from build123d import *

# Parameters (mm, degrees)
EXTRUDE_1_DEPTH = 75
CHAMFER_1_SIZE  = 15
CHAMFER_2_SIZE  = 3


with BuildPart() as part:
    # 草图1 → 凸台-拉伸1 (new body)
    with BuildSketch(Plane.XY):
        Polygon((0, 0), (70, 0), (70, 5), (40, 5), (40, 55), (37, 55), (37, 5), (35.2, 5), (35.2, 55), (32.2, 55), (32.2, 5), (0, 5), align=None)
    extrude(amount=EXTRUDE_1_DEPTH)

    # 倒角1
    chamfer_1_edges = [part.edges().sort_by_distance(p)[0] for p in [
        (32.2, 5, 37.5),
        (40, 5, 37.5),
    ]]
    chamfer(chamfer_1_edges, length=CHAMFER_1_SIZE)

    # 倒角2
    chamfer_2_edges = [part.edges().sort_by_distance(p)[0] for p in [
        (37, 55, 37.5),
        (35.2, 55, 37.5),
    ]]
    chamfer(chamfer_2_edges, length=CHAMFER_2_SIZE - 0.0001)  # a hair under: the kernel refuses the full size


solid = part.part
CAD build for the part. Positions are in the model's coordinates, mm. A direction names the side the tool comes from. Coordinates: 2 decimals unless noted, no trailing zeros. Write each loop counter-clockwise with the first axis right and the second up, starting at its lowest first coordinate (ties: lowest second). Pieces come first, ordered by that corner, then holes. Notation, with made-up numbers: M 23.5,-2.75 L 56.5,-2.75 A30 ccw 56.5,24.25 Z; hole C -35.5,-12.5 d11. An arc over 180 degrees is marked long. Answer as a JSON object with one key per item and string values. Group by question number.
1) Saw through at C-C (x = 62.5). Write the cut outline in (y, z).
2) Mould opens along X. For faces 1 (the face through (0, 3, 37)), 2 (the face through (35.2, 28, 37)), 3 (the face through (35, 17, 75)), 4 (the face through (37, 29, 37)) say: +X half, -X half, draft (parallel to the pull), parting line (faces both ways), or undercut.
3) Saw through at A-A (y = 15.5). Write the cut outline in (x, z), plus the area to 4 significant figures.
4) Pin check, flat tips, straight feed: pin 1 Ø4 at (x, z) = (28.5, 31) entering from +Y; pin 2 Ø5 at (x, z) = (6.5, 49.5) entering from +Y; pin 3 Ø3 at (y, z) = (44, 12.5) entering from +X. Stop position of each tip, or through.
5) Saw through at D-D (y = 6). Write the cut outline in (x, z).
6) Tool access for faces 5 (the face through (32.2, 38, 37)), 6 (the face through (33.7, 53.5, 37)), 7 (the face through (35, 17, 0)), 8 (the face through (40, 37, 37)), 9 (the face through (35, 0, 37)): list every direction of +Z, -Z, +X, -X, +Y, -Y with a clear straight run to the whole face (end or side of a thin tool).
7) Wall check: line 1 (X direction, y = 43, z = 9.5); line 2 (X direction, y = 14, z = 70); line 3 (Y direction, x = 9.5, z = 58.5). Give the ranges that are in metal, low to high. Write a range as from..to.
Values follow:
{
 "1": {"outline": "M 0,0 L 5,0 L 5,75 L 0,75 Z"},
 "2": {"face 1": "-X half", "face 2": "undercut", "face 3": "draft", "face 4": "undercut"},
 "3": {"outline": "M 27.7,0 L 35.2,0 L 35.2,75 L 27.7,75 Z; M 37,0 L 44.5,0 L 44.5,75 L 37,75 Z", "area": "1,125 mm2"},
 "4": {"pin 1": "stops at y = 18.3", "pin 2": "stops at y = 5", "pin 3": "stops at x = 40"},
 "5": {"outline": "M 18.2,0 L 35.2,0 L 35.2,75 L 18.2,75 Z; M 37,0 L 54,0 L 54,75 L 37,75 Z"},
 "6": {"face 5": "+Z, -Z, -X, +Y", "face 6": "+Z, -Z, +Y", "face 7": "-Z, +X, -X, +Y, -Y", "face 8": "+Z, -Z, +X, +Y", "face 9": "+Z, -Z, +X, -X, -Y"},
 "7": {"line 1": "x = 32.2..35.2, 37..40", "line 2": "x = 26.2..35.2, 37..46", "line 3": "y = 0..5"}
}
